```python
from build123d import *

# Parameters (mm, degrees)
SKETCH1_W           = 5.4
SKETCH1_H           = 48.265
BOSS_EXTRUDE1_DEPTH = 5.4
SKETCH2_W           = 5.31872
SKETCH2_H           = 48.18372
BOSS_EXTRUDE2_DEPTH = 5.4


with BuildPart() as part:
    # Sketch1 → Boss-Extrude1 (new body)
    with BuildSketch(Plane.XY):
        Polygon((-181.028382108, -13.967555325), (-181.028382108, -8.567555325), (-200.453382108, -8.567555325), (-200.453382108, -13.967555325), (-219.878382108, -13.967555325), (-219.878382108, -8.567555325), (-239.303382108, -8.567555325), (-239.303382108, -13.967555325), (-244.703382108, -13.967555325), (-244.703382108, -62.232555325), (-239.303382108, -62.232555325), (-239.303382108, -110.497555325), (-244.703382108, -110.497555325), (-244.703382108, -158.762555325), (-239.303382108, -158.762555325), (-239.303382108, -207.027555325), (-244.703382109, -207.027555325), (-244.703382109, -255.292555325), (-239.303382108, -255.292555325), (-239.303382108, -260.692555325), (-219.878382108, -260.692555325), (-219.878382108, -255.292555325), (-200.453382108, -255.292555325), (-200.453382108, -260.692555325), (-181.028382108, -260.692555325), (-181.028382108, -255.292555325), (-161.603382108, -255.292555325), (-161.603382108, -260.692555325), (-142.178382108, -260.692555325), (-142.178382108, -255.292555325), (-122.753382108, -255.292555325), (-122.753382108, -260.692555325), (-103.328382108, -260.692555325), (-103.328382108, -255.292555325), (-83.903382108, -255.292555325), (-83.903382108, -260.692555325), (-64.478382108, -260.692555325), (-64.478382108, -255.292555325), (-45.053382108, -255.292555325), (-45.053382108, -260.692555325), (-25.628382108, -260.692555325), (-25.628382108, -255.292555325), (-6.203382108, -255.292555325), (-6.203382108, -260.692555325), (13.221617892, -260.692555325), (13.221617892, -255.292555325), (32.646617892, -255.292555325), (32.646617892, -260.692555325), (52.071617892, -260.692555325), (52.071617892, -207.027555325), (57.471617892, -207.027555325), (57.471617892, -158.762555325), (52.071617892, -158.762555325), (52.071617892, -110.497555325), (57.471617892, -110.497555325), (57.471617892, -62.232555325), (52.071617892, -62.232555325), (52.071617892, -8.567555325), (32.646617892, -8.567555325), (32.646617892, -13.967555325), (13.221617892, -13.967555325), (13.221617892, -8.567555325), (-6.203382108, -8.567555325), (-6.203382108, -13.967555325), (-25.628382108, -13.967555325), (-25.628382108, -8.567555325), (-45.053382108, -8.567555325), (-45.053382108, -13.967555325), (-64.478382108, -13.967555325), (-64.478382108, -8.567555325), (-83.903382108, -8.567555325), (-83.903382108, -13.967555325), (-103.328382108, -13.967555325), (-103.328382108, -8.567555325), (-122.753382108, -8.567555325), (-122.753382108, -13.967555325), (-142.178382108, -13.967555325), (-142.178382108, -8.567555325), (-161.603382108, -8.567555325), (-161.603382108, -13.967555325), align=None)
        with Locations((-100.653382108, -182.895055325)):
            Rectangle(SKETCH1_W, SKETCH1_H, mode=Mode.SUBTRACT)
        with Locations((-100.653382108, -86.365055325)):
            Rectangle(SKETCH1_W, SKETCH1_H, mode=Mode.SUBTRACT)
    extrude(amount=BOSS_EXTRUDE1_DEPTH)

    # Sketch2 → Boss-Extrude2 (add)
    with BuildSketch(Plane.XY.offset(5.4)):
        Polygon((-239.344022108, -8.526915325), (-239.344022108, -13.926915325), (-244.744022108, -13.926915325), (-244.744022108, -62.273195325), (-239.344022108, -62.273195325), (-239.344022108, -110.456915325), (-244.744022108, -110.456915325), (-244.744022108, -158.803195325), (-239.344022108, -158.803195325), (-239.344022108, -206.986915325), (-244.744022109, -206.986915325), (-244.744022109, -255.333195325), (-239.344022108, -255.333195325), (-239.344022108, -260.733195325), (-219.837742108, -260.733195325), (-219.837742108, -255.333195325), (-200.494022108, -255.333195325), (-200.494022108, -260.733195325), (-180.987742108, -260.733195325), (-180.987742108, -255.333195325), (-161.644022108, -255.333195325), (-161.644022108, -260.733195325), (-142.137742108, -260.733195325), (-142.137742108, -255.333195325), (-122.794022108, -255.333195325), (-122.794022108, -260.733195325), (-103.287742108, -260.733195325), (-103.287742108, -255.333195325), (-83.944022108, -255.333195325), (-83.944022108, -260.733195325), (-64.437742108, -260.733195325), (-64.437742108, -255.333195325), (-45.094022108, -255.333195325), (-45.094022108, -260.733195325), (-25.587742108, -260.733195325), (-25.587742108, -255.333195325), (-6.244022108, -255.333195325), (-6.244022108, -260.733195325), (13.262257892, -260.733195325), (13.262257892, -255.333195325), (32.605977892, -255.333195325), (32.605977892, -260.733195325), (52.112257892, -260.733195325), (52.112257892, -207.068195325), (57.512257892, -207.068195325), (57.512257892, -158.721915325), (52.112257892, -158.721915325), (52.112257892, -110.538195325), (57.512257892, -110.538195325), (57.512257892, -62.191915325), (52.112257892, -62.191915325), (52.112257892, -8.526915325), (32.605977892, -8.526915325), (32.605977892, -13.926915325), (13.262257892, -13.926915325), (13.262257892, -8.526915325), (-6.244022108, -8.526915325), (-6.244022108, -13.926915325), (-25.587742108, -13.926915325), (-25.587742108, -8.526915325), (-45.094022108, -8.526915325), (-45.094022108, -13.926915325), (-64.437742108, -13.926915325), (-64.437742108, -8.526915325), (-83.944022108, -8.526915325), (-83.944022108, -13.926915325), (-103.287742108, -13.926915325), (-103.287742108, -8.526915325), (-122.794022108, -8.526915325), (-122.794022108, -13.926915325), (-142.137742108, -13.926915325), (-142.137742108, -8.526915325), (-161.644022108, -8.526915325), (-161.644022108, -13.926915325), (-180.987742108, -13.926915325), (-180.987742108, -8.526915325), (-200.494022108, -8.526915325), (-200.494022108, -13.926915325), (-219.837742108, -13.926915325), (-219.837742108, -8.526915325), align=None)
        with Locations((-100.653382108, -86.365055325)):
            Rectangle(SKETCH2_W, SKETCH2_H, mode=Mode.SUBTRACT)
        with Locations((-100.653382108, -182.895055325)):
            Rectangle(SKETCH2_W, SKETCH2_H, mode=Mode.SUBTRACT)
    extrude(amount=-BOSS_EXTRUDE2_DEPTH)


solid = part.part
```
Design review of the part built by this model. Coordinates are the model's own, in mm. Coordinates: 2 decimals unless noted, no trailing zeros. Loops run counter-clockwise (first coordinate to the right, second up) from the corner with the lowest first, then second, coordinate; pieces in that order, holes last. Notation, with made-up numbers: M 45,79 L 74,79 A16 cw 74,107 Z; hole C -4.75,59 d2. An arc over 180 degrees is marked long. One line per question, with ' | ' between items.
(1) We need section C-C (x = -207). Give the boundary of the cut face in (y, z), and give its area (3 significant figures).
Filled in:
outline: M -255.33,0 L -13.93,0 L -13.93,5.4 L -255.33,5.4 Z | area: 1,300 mm^2
(2) We need section B-B (z = 1). Count the separate pieces of the cut face and the enclosed holes in it, and give its area (3 significant figures).
Filled in:
separate pieces: 1 | enclosed holes: 2 | area: 72,800 mm^2
(3) For pin 1 Ø2 at (x, z) = (-174.5, 2.5) entering from -Y; pin 2 Ø2.5 at (y, z) = (-12, 2) entering from +X; pin 3 Ø2.5 at (y, z) = (-10, 4) entering from -X; pin 4 Ø1.5 at (x, y) = (-143.5, -156) entering from -Z, all flat-tipped, find the tip position at first contact; note any pin that passes through.
Filled in:
pin 1: stops at y = -255.33 | pin 2: stops at x = 52.11 | pin 3: stops at x = -239.34 | pin 4: stops at z = 0
(4) We need section A-A (y = -180.5). Give the boundary of the cut face in (x, z).
Filled in:
outline: M -239.34,0 L -103.31,0 L -103.31,5.4 L -239.34,5.4 Z; M -97.99,0 L 57.51,0 L 57.51,5.4 L -97.99,5.4 Z
(5) We need section D-D (y = -148.5). Give the boundary of the cut face in (x, z).
Filled in:
outline: M -244.74,0 L 52.11,0 L 52.11,5.4 L -244.74,5.4 Z
(6) Wall thickness on probe 1 along X at (y, z) = (-83, 2.6); probe 2 along Y at (x, z) = (-124, 3); probe 3 along X at (y, z) = (-238.5, 4.85): over which ranges is each line inside the solid? List them lowest first.
Filled in:
probe 1: x = -239.34 to -103.31, -97.99 to 57.51 | probe 2: y = -255.33 to -13.93 | probe 3: x = -244.74 to 52.11
